Autodesk Inventor part; units mm, degrees
ref_plane "YZ Plane" through (0, 0, 0) normal (1, 0, 0) x (0, 1, 0)
ref_plane "XZ Plane" through (0, 0, 0) normal (0, 1, 0) x (-1, 0, 0)
ref_plane "XY Plane" through (0, 0, 0) normal (0, 0, 1) x (1, 0, 0)
sketch "Sketch1" plane through (0, 0, 0) normal (0, 1, 0) x (-1, 0, 0)
  line L0 (0, 0) -> (100, 0)
  line L1 (100, 0) -> (100, -180)
  line L2 (100, -180) -> (0, -180)
  line L3 (0, -180) -> (0, 0)
  dimension "d0" = 100
  dimension "d1" = 180
extrude "Extrusion1" add sketch "Sketch1" along normal blind 5
sketch "Sketch2" plane through (0, 5, 0) normal (0, 1, 0) x (1, 0, 0)
  line L0 (0, 160) -> (-100, 160)
  line L1 (-100, 160) -> (-100, 155)
  line L2 (-100, 155) -> (0, 155)
  line L3 (0, 155) -> (0, 160)
  line L4 (0, 180) -> (-100, 180)
  point P0 (0, 0)
  dimension "d4" = 100
  dimension "d5" = 5
  dimension "d6" = 20
extrude "Extrusion2" add sketch "Sketch2" along normal blind 95
sketch "Sketch5" plane through (0, 5, -160) normal (0, 0, -1) x (-1, 0, 0)
  line L0 (28, 87) -> (52, 87)
  line L1 (52, 87) -> (52, 53)
  line L2 (52, 53) -> (28, 53)
  line L3 (28, 53) -> (28, 87)
  line L4 (28, 87) -> (52, 53) construction
  line L5 (52, 87) -> (28, 53) construction
  line L6 (0, 0) -> (0, 95)
  line L7 (0, 95) -> (100, 95)
  circle A0 centre (28, 87) radius 2
  circle A1 centre (52, 87) radius 2
  circle A2 centre (28, 53) radius 2
  circle A3 centre (52, 53) radius 2
  point P0 (0, -5)
  point P1 (40, 70)
  point P2 (50, 95)
  dimension "d14" = 24
  dimension "d15" = 34
  dimension "d16" = 40
  dimension "d17" = 25
  dimension "d19" = 4
  dimension "d20" = 4
  dimension "d21" = 4
  dimension "d22" = 4
extrude "Extrusion4" cut sketch "Sketch5" against normal blind 95 contours L3 A0 L0 | L0 A0 L3 | A1 L1 L0 | L0 L1 A1 | A2 L2 L3 | L3 L2 A2 | A3 L2 L1 | L1 L2 A3
sketch "Sketch12" plane through (0, 5, -160) normal (0, 0, -1) x (-1, 0, 0)
  line L0 (0, 95) -> (100, 95)
  line L1 (100, 95) -> (60, 95)
  line L2 (100, 0) -> (0, 0)
  line L3 (60, 95) -> (100, 0)
  line L4 (100, 0) -> (100, 95)
  point P0 (0, -5)
  dimension "d72" = 40
extrude "Extrusion10" cut sketch "Sketch12" against normal blind 14
sketch "Sketch13" plane through (0, 5, 0) normal (0, 1, 0) x (1, 0, 0)
  line L0 (-20, 23) -> (-60, 23)
  line L1 (-60, 23) -> (-60, 3)
  line L2 (-60, 3) -> (-20, 3)
  line L3 (-20, 3) -> (-20, 23)
  line L4 (-20, 23) -> (-60, 3) construction
  line L5 (-60, 23) -> (-20, 3) construction
  line L6 (-100, 0) -> (0, 0)
  line L7 (0, 0) -> (0, 155)
  line L8 (-20, 88) -> (-60, 88)
  line L9 (-60, 88) -> (-60, 68)
  line L10 (-60, 68) -> (-20, 68)
  line L11 (-20, 68) -> (-20, 88)
  line L12 (-20, 88) -> (-60, 68) construction
  line L13 (-60, 88) -> (-20, 68) construction
  point P0 (-40, 13)
  point P1 (-40, 78)
  dimension "d76" = 40
  dimension "d77" = 20
  dimension "d78" = 3
  dimension "d79" = 40
  dimension "d80" = 40
  dimension "d81" = 20
  dimension "d82" = 45
  dimension "d83" = 40
extrude "Extrusion11" add sketch "Sketch13" along normal blind 38
sketch "Sketch14" plane through (0, 43, 0) normal (0, 1, 0) x (1, 0, 0)
  line L0 (-4, 90.5) -> (-76, 90.5)
  line L1 (-76, 90.5) -> (-76, 65.5)
  line L2 (-76, 65.5) -> (-4, 65.5)
  line L3 (-4, 65.5) -> (-4, 90.5)
  line L4 (-4, 90.5) -> (-76, 65.5) construction
  line L5 (-76, 90.5) -> (-4, 65.5) construction
  line L6 (-20, 88) -> (-60, 88)
  line L7 (-20, 68) -> (-20, 88)
  line L8 (-4, 25.5) -> (-76, 25.5)
  line L9 (-76, 25.5) -> (-76, 0.5)
  line L10 (-76, 0.5) -> (-4, 0.5)
  line L11 (-4, 0.5) -> (-4, 25.5)
  line L12 (-4, 25.5) -> (-76, 0.5) construction
  line L13 (-76, 25.5) -> (-4, 0.5) construction
  line L14 (-20, 23) -> (-60, 23)
  line L15 (-20, 3) -> (-20, 23)
  point P0 (0, 0)
  point P1 (-40, 78)
  point P2 (-40, 13)
  dimension "d86" = 72
  dimension "d87" = 25
  dimension "d88" = 10
  dimension "d89" = 20
  dimension "d90" = 72
  dimension "d91" = 25
  dimension "d92" = 10
  dimension "d93" = 20
extrude "Extrusion12" add sketch "Sketch14" along normal blind 14
sketch "Sketch16" plane through (0, 5, 0) normal (0, 1, 0) x (1, 0, 0)
  line L0 (0, 180) -> (-100, 180)
  line L1 (-38, 160) -> (-43, 160)
  line L2 (-43, 160) -> (-43, 180)
  line L3 (-43, 180) -> (-38, 180)
  line L4 (-38, 180) -> (-38, 160)
  line L5 (0, 160) -> (0, 180)
  point P0 (0, 0)
  dimension "d96" = 20
  dimension "d97" = 38
  dimension "d98" = 5
extrude "Extrusion13" add sketch "Sketch16" along normal blind 95
sketch "Sketch18" plane through (0, 5, 0) normal (0, 1, 0) x (1, 0, 0)
  line L0 (-60, 155) -> (-100, 155)
  line L1 (-82, 155) -> (-77, 155)
  line L2 (-77, 155) -> (-77, 125)
  line L3 (-77, 125) -> (-82, 125)
  line L4 (-82, 125) -> (-82, 155)
  line L5 (-23, 155) -> (-18, 155)
  line L6 (-18, 155) -> (-18, 125)
  line L7 (-18, 125) -> (-23, 125)
  line L8 (-23, 125) -> (-23, 155)
  line L9 (-100, 155) -> (-100, 0)
  line L10 (0, 0) -> (0, 155)
  dimension "d103" = 5
  dimension "d104" = 30
  dimension "d105" = 5
  dimension "d106" = 30
  dimension "d107" = 18
  dimension "d108" = 18
extrude "Extrusion15" add sketch "Sketch18" along normal blind 40
sketch "Sketch20" plane through (-43, 5, -180) normal (-1, 0, 0) x (0, 0, 1)
  line L0 (20, 0) -> (20, 95)
  line L1 (20, 95) -> (20, 65)
  line L2 (20, 65) -> (15, 65)
  line L3 (0, 0) -> (20, 0)
  line L4 (15, 65) -> (0, 0)
  line L5 (0, 95) -> (20, 95)
  line L6 (0, 0) -> (0, 95)
  line L7 (0, 95) -> (20, 95)
  point P0 (180, -5)
  dimension "d114" = 30
  dimension "d115" = 5
extrude "Extrusion17" cut sketch "Sketch20" against normal blind 10 contours L2 L4 L6 L5 L0
sketch "Sketch21" plane through (0, 5, 0) normal (0, 1, 0) x (1, 0, 0)
  circle A0 centre (-90, 10) radius 2.5
  line L0 (-100, 155) -> (-100, 0)
  line L1 (-100, 0) -> (0, 0)
  circle A1 centre (-10, 10) radius 2.5
  line L2 (0, 0) -> (0, 155)
  circle A2 centre (-90, 170) radius 2.5
  line L3 (-43, 180) -> (-100, 180)
  line L4 (-100, 180) -> (-100, 160)
  circle A3 centre (-10, 170) radius 2.5
  line L5 (0, 180) -> (-38, 180)
  line L6 (0, 160) -> (0, 180)
  circle A4 centre (-50, 50) radius 2.5
  circle A5 centre (-50, 130) radius 2.5
  dimension "d118" = 5
  dimension "d119" = 10
  dimension "d120" = 10
  dimension "d121" = 5
  dimension "d122" = 10
  dimension "d123" = 10
  dimension "d124" = 5
  dimension "d125" = 10
  dimension "d126" = 10
  dimension "d127" = 5
  dimension "d128" = 10
  dimension "d129" = 10
  dimension "d130" = 5
  dimension "d131" = 5
  dimension "d132" = 50
  dimension "d133" = 50
extrude "Extrusion18" cut sketch "Sketch21" against normal blind 10
sketch "Sketch27" plane through (0, 57, 0) normal (0, 1, 0) x (1, 0, 0)
  circle A0 centre (-66.5, 78) radius 2.5
  line L0 (-4, 90.5) -> (-76, 90.5)
  line L1 (-76, 90.5) -> (-76, 65.5)
  circle A1 centre (-13.5, 78) radius 2.5
  line L2 (-76, 65.5) -> (-4, 65.5)
  circle A2 centre (-66.5, 13) radius 2.5
  line L3 (-76, 25.5) -> (-76, 0.5)
  line L4 (-76, 0.5) -> (-4, 0.5)
  circle A3 centre (-13.5, 13) radius 2.5
  line L5 (-4, 0.5) -> (-4, 25.5)
  point P0 (0, 0)
  dimension "d137" = 5
  dimension "d138" = 12.5
  dimension "d139" = 9.5
  dimension "d140" = 5
  dimension "d141" = 53
  dimension "d142" = 12.5
  dimension "d143" = 5
  dimension "d144" = 9.5
  dimension "d145" = 12.5
  dimension "d146" = 5
  dimension "d147" = 9.5
  dimension "d148" = 12.5
extrude "Extrusion19" cut sketch "Sketch27" against normal blind 15
sketch "Sketch28" plane through (-82, 5, -155) normal (-1, 0, 0) x (0, 0, 1)
  line L0 (0, 40) -> (30, 40)
  line L1 (30, 40) -> (10, 40)
  line L2 (30, 0) -> (30, 40)
  line L3 (10, 40) -> (30, 0)
  line L4 (30, 0) -> (30, 40)
  point P0 (155, -5)
  dimension "d151" = 20
extrude "Extrusion20" cut sketch "Sketch28" against normal blind 200
sketch "Sketch29" plane through (0, 0, 0) normal (0, -1, 0) x (1, 0, 0)
  circle A0 centre (-90, -90) radius 2.5
  line L0 (-100, 0) -> (-100, -180)
  line L1 (0, 0) -> (-100, 0)
  circle A1 centre (-10, -90) radius 2.5
  line L2 (0, -180) -> (0, 0)
  dimension "d154" = 5
  dimension "d155" = 10
  dimension "d156" = 90
  dimension "d157" = 5
  dimension "d158" = 10
  dimension "d159" = 90
extrude "Extrusion21" cut sketch "Sketch29" against normal blind 5
sketch "Sketch30" plane through (0, 0, 0) normal (0, -1, 0) x (1, 0, 0)
  circle A0 centre (-50, -130) radius 2.5
  circle A1 centre (-50, -130) radius 2.5
  circle A2 centre (-50, -50) radius 2.5
  circle A3 centre (-50, -50) radius 2.5
  point P0 (0, 0)
  dimension "d162" = 5
  dimension "d163" = 5
extrude "Extrusion22" add sketch "Sketch30" against normal blind 5
properties part number "Giá đỡ động cơ"
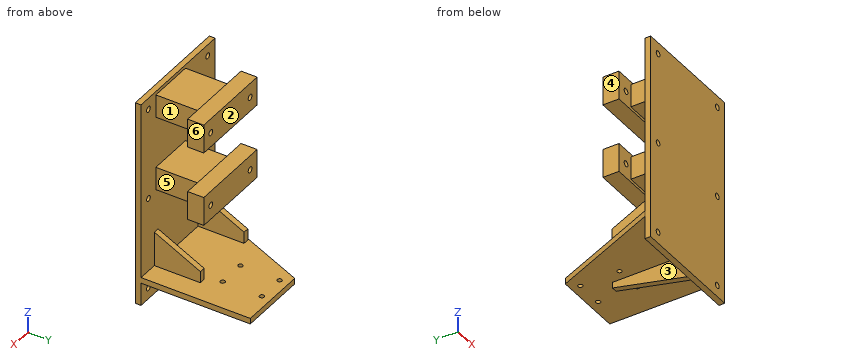
Source: CAD feature listing. Evaluate the final solid. Frame: model axes, mm. Face numbers are marked on the shaded views. A direction names the side the tool comes from. Coordinates: 2 decimals unless noted, no trailing zeros. Loops run counter-clockwise (first coordinate to the right, second up) from the corner with the lowest first, then second, coordinate; pieces in that order, holes last. Notation, with made-up numbers: (61, 45) - (78, 45) arc R20 cw to (78, 83) - close; hole circle Ø1 at (52, 45.5). An arc over 180 degrees is marked (long way). One line per question, with ' | ' between items.
1) Section C-C, the plane z = -150. Return loops of the section in (x, y), then the cut area to 3 significant figures.
Report:
outline: (-100, 0) - (0, 0) - (0, 5) - (-18, 5) - (-18, 45) - (-23, 45) - (-23, 5) - (-77, 5) - (-77, 45) - (-82, 45) - (-82, 5) - (-100, 5) - close | area: 900 mm²
2) Section A-A, the plane x = -90. Return loops of the section in (y, z).
Report:
outline: (0, -180) - (5, -180) - (5, -172.5) - (0, -172.5) - close; (0, -167.5) - (5, -167.5) - (5, -160) - (28.75, -160) - (28.75, -155) - (5, -155) - (5, -92.5) - (0, -92.5) - close; (0, -87.5) - (5, -87.5) - (5, -12.5) - (0, -12.5) - close; (0, -7.5) - (5, -7.5) - (5, 0) - (0, 0) - close
3) Set-up query: the marked faces 4, 5 and 6. Return all of +Z, -Z, +X, -X, +Y, -Y with unobstructed straight access to the full face (end or side cutting, diameter ignored); none if empty.
Report:
face 4: +Z, -X, +Y | face 5: +Z, +X | face 6: +Z, +X, +Y
4) First-contact query: P1, Ø6, axis at x = -53, z = -147.5, coming from the +Y side; P2, Ø2.5, axis at x = -52, y = 92, coming from the +Z side; P3, Ø10, axis at y = 15, z = -14.5, coming from the +X side; P4, Ø19, axis at x = -32, y = 24, coming from the -Z side. Flat tips, straight axial feed; report the tip coordinate or a pass-through.
Report:
P1: stops at y = 5 | P2: passes through | P3: stops at x = -20 | P4: stops at z = -177.32
5) Line query: line 1 along Y through (x, z) = (-28, -157); line 2 along Z through (x, y) = (-13.5, 48); line 3 along Z through (x, y) = (-10, 3). Output: solid intervals per line, ascending.
Report:
line 1: y = 0 to 56, 60 to 90, 94 to 100 | line 2: z = -160 to -155, -90.5 to -80.5, -75.5 to -65.5, -25.5 to -15.5, -10.5 to -0.5 | line 3: z = -180 to -172.5, -167.5 to -92.5, -87.5 to -12.5, -7.5 to 0
6) Pull-direction query (Y, two-part tool) for the marked faces 1, 2 and 3; classes: released by +Y, released by -Y, zero draft, split by the parting line, or undercut.
Report:
face 1: undercut | face 2: released by +Y | face 3: zero draft
7) Section D-D, the plane y = 92. Return loops of the section in (x, z).
Report:
outline: (-63.37, -160) - (-54, -160) - (-54, -155) - (-63.37, -155) - close; (-50, -160) - (-30, -160) - (-30, -155) - (-50, -155) - close; (-26, -160) - (0, -160) - (0, -155) - (-26, -155) - close
8) Section B-B, the plane z = -170. Return loops of the section in (x, y), then the cut area to 3 significant figures.
Report:
outline: (-100, 0) - (-92.5, 0) - (-92.5, 5) - (-100, 5) - close; (-87.5, 0) - (-12.5, 0) - (-12.5, 5) - (-38, 5) - (-38, 48.33) - (-43, 48.33) - (-43, 5) - (-87.5, 5) - close; (-7.5, 0) - (0, 0) - (0, 5) - (-7.5, 5) - close | area: 667 mm²
